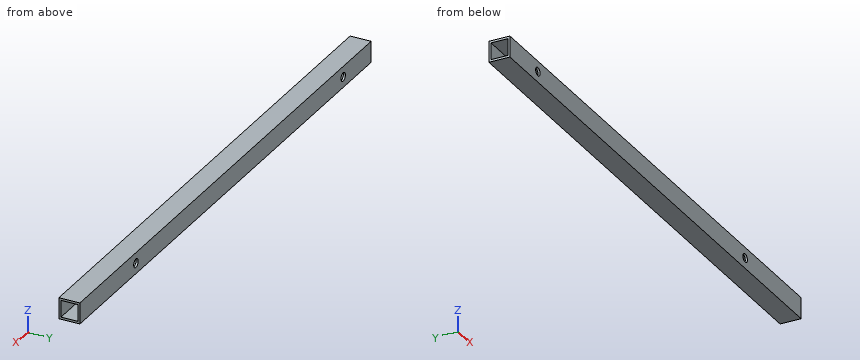
```python
from build123d import *

# Parameters (mm, degrees)
SKETCH1_W           = 3.96875
SKETCH1_H           = 3.96875
BOSS_EXTRUDE1_DEPTH = 104
SKETCH2_W           = 3.175
SKETCH2_H           = 3.175
CUT_EXTRUDE1_DEPTH  = 105.037856035
SKETCH3_R           = 0.79375
CUT_EXTRUDE2_DEPTH  = 105.094614273
SKETCH4_R           = 0.79375
CUT_EXTRUDE3_DEPTH  = 105.094614273


with BuildPart() as part:
    # Sketch1 → Boss-Extrude1 (new body)
    with BuildSketch(Plane(origin=(0, 0, 0), x_dir=(0, 0, -1), z_dir=(1, 0, 0))):
        Rectangle(SKETCH1_W, SKETCH1_H)
    extrude(amount=BOSS_EXTRUDE1_DEPTH)

    # Sketch2 → Cut-Extrude1 (cut, through all)
    with BuildSketch(Plane.ZY):
        Rectangle(SKETCH2_W, SKETCH2_H)
    extrude(amount=-CUT_EXTRUDE1_DEPTH, mode=Mode.SUBTRACT)

    # Sketch3 → Cut-Extrude2 (cut, through all)
    with BuildSketch(Plane(origin=(0, 1.984375, 0), x_dir=(1, 0, 0), z_dir=(0, 1, 0))):
        with Locations(Location((10, 0, 0), (0, 0, 270))):
            Circle(SKETCH3_R)
    extrude(amount=-CUT_EXTRUDE2_DEPTH, mode=Mode.SUBTRACT)

    # Sketch4 → Cut-Extrude3 (cut, through all)
    with BuildSketch(Plane(origin=(0, 1.984375, 0), x_dir=(1, 0, 0), z_dir=(0, 1, 0))):
        with Locations(Location((84, 0, 0), (0, 0, 270))):
            Circle(SKETCH4_R)
    extrude(amount=-CUT_EXTRUDE3_DEPTH, mode=Mode.SUBTRACT)


solid = part.part
```
Verification items for the finished model (mm, model axes). Coordinates: 2 decimals unless noted, no trailing zeros. Order: outer loops, then holes, each group sorted by start corner. A loop starts at its lowest first (then second) coordinate and runs counter-clockwise, first axis right, second up. Notation, with made-up numbers: (-26, 20.25) - (31, 20.25) arc R20 cw to (31, 48.25) - close; hole circle Ø6 at (48, 11). An arc over 180 degrees is marked (long way). Return JSON: item names as keys, results as strings.
(1) Section check A-A, the plane y = -0.45. Record the cut outline in (x, z).
Filled sheet:
{"outline": "(0, -1.98) - (104, -1.98) - (104, -1.59) - (0, -1.59) - close; (0, 1.59) - (104, 1.59) - (104, 1.98) - (0, 1.98) - close"}
(2) Thickness scan on line 1 along X through (y, z) = (-1.65, 0); line 2 along Y through (x, z) = (57, -0.35); line 3 along Z through (x, y) = (84, -1.8). Record the ranges inside material, lowest first.
Filled sheet:
{"line 1": "x = 0 to 9.21, 10.79 to 83.21, 84.79 to 104", "line 2": "y = -1.98 to -1.59, 1.59 to 1.98", "line 3": "z = -1.98 to -0.79, 0.79 to 1.98"}
(3) Section check B-B, the plane x = 75. Record the cut outline in (y, z), and give its area (3 significant figures).
Filled sheet:
{"outline": "(-1.98, -1.98) - (1.98, -1.98) - (1.98, 1.98) - (-1.98, 1.98) - close; hole (-1.59, -1.59) - (1.59, -1.59) - (1.59, 1.59) - (-1.59, 1.59) - close", "area": "5.67 mm^2"}
